from build123d import *

# Parameters (mm, degrees)
ESQUISSE2_R                  = 14.25
BOSS_EXTRU_1_DEPTH           = 3.25
ESQUISSE3_R                  = 1.2
ENL_V_MAT_EXTRU_1_DEPTH      = 4.25
ESQUISSE10_R                 = 1.7
ENL_V_MAT_EXTRU_2_DEPTH      = 1
ENL_V_MAT_EXTRU_2_DEPTH_BACK = 7.5
ESQUISSE17_R                 = 4
ENL_V_MAT_EXTRU_8_DEPTH      = 2
ESQUISSE13_R                 = 1
ENL_V_MAT_EXTRU_4_DEPTH      = 35.402543264


with BuildPart() as part:
    # Esquisse2 → Boss.-Extru.1 (new body, symmetric)
    with BuildSketch(Plane.XY):
        Circle(ESQUISSE2_R)
    extrude(amount=BOSS_EXTRU_1_DEPTH, both=True)

    # Esquisse3 → Enlèv. mat.-Extru.1 (cut, through all)
    with BuildSketch(Plane.XY):
        with Locations((0, 8.25)):
            Circle(ESQUISSE3_R)
        with Locations((-8.25, 0)):
            Circle(ESQUISSE3_R)
        with Locations((0, -8.25)):
            Circle(ESQUISSE3_R)
        with Locations((8.25, 0)):
            Circle(ESQUISSE3_R)
    extrude(amount=ENL_V_MAT_EXTRU_1_DEPTH, mode=Mode.SUBTRACT)

    # Esquisse10 → Enlèv. mat.-Extru.2 (cut, two sides)
    with BuildSketch(Plane(origin=(0, 0, -3.25), x_dir=(-1, 0, 0), z_dir=(0, 0, -1))) as enl_v_mat_extru_2_sk:
        with Locations((-8.25, 0)):
            Circle(ESQUISSE10_R)
        with Locations((0, 8.25)):
            Circle(ESQUISSE10_R)
        with Locations((8.25, 0)):
            Circle(ESQUISSE10_R)
        with Locations((0, -8.25)):
            Circle(ESQUISSE10_R)
    extrude(amount=ENL_V_MAT_EXTRU_2_DEPTH, mode=Mode.SUBTRACT)
    extrude(enl_v_mat_extru_2_sk.sketch, amount=-ENL_V_MAT_EXTRU_2_DEPTH_BACK, mode=Mode.SUBTRACT)

    # Esquisse17 → Enlèv. mat.-Extru.8 (cut)
    with BuildSketch(Plane.XY.offset(3.25)):
        Circle(ESQUISSE17_R)
    extrude(amount=-ENL_V_MAT_EXTRU_8_DEPTH, mode=Mode.SUBTRACT)

    # Esquisse13 → Enlèv. mat.-Extru.4 (cut, through all)
    with BuildSketch(Plane(origin=(10.076271632, -10.076271632, 0), x_dir=(-0.707106781, -0.707106781, 0), z_dir=(0.707106781, -0.707106781, 0))):
        Circle(ESQUISSE13_R)
    extrude(amount=-ENL_V_MAT_EXTRU_4_DEPTH, mode=Mode.SUBTRACT)

    # Esquisse18 → Enlèvement de matière-Révolution1 (revolve, cut)
    with BuildSketch(Plane(origin=(0, 0, 0), x_dir=(1, 0, 0), z_dir=(0, 1, 0))):
        Polygon((14.25, 2.5), (12.806624327, 0), (14.25, -2.5), align=None)
    revolve(axis=Axis((0, 0, -3.25), (0, 0, 1)), mode=Mode.SUBTRACT)


solid = part.part
Design review of the part built by this model. Coordinates are the model's own, in mm. A direction names the side the tool comes from. Give positions to 0.01 mm unless a question says otherwise; leave off trailing zeros. Order: outer loops, then holes, each group sorted by start corner. A loop starts at its lowest first (then second) coordinate and runs counter-clockwise, first axis right, second up.
1. Mouldability with a two-part tool opening along Y and no side actions: class faces 1 (the cylindrical face through (13.163, -5.458, 2.88)), 2 (the cylindrical face through (0.37, 6.59, -0.05)), 3 (the cylindrical face through (-0.54, -0.81, -0.3)), 4 (the flat face through (0, 0, -3.25)) as +Y half, -Y half, draft (parallel to the pull), parting line (faces both ways), or undercut.
Solution:
face 1: parting line
face 2: undercut
face 3: undercut
face 4: draft
2. To check wall thickness, follow L1, parallel to Y at x = 0, z = 2.65; L2, parallel to Y at x = -8.5, z = 0.5; L3, parallel to Y at x = -9, z = 1.5. State the ranges of each line that lie inside material, in increasing order.
Solution:
L1: y = -14.25 to -9.95, -6.55 to -4, 4 to 6.55, 9.95 to 14.25
L2: y = -9.96 to -1.68, 1.68 to 7.28, 9.72 to 9.96
L3: y = -10.29 to -1.53, 1.53 to 10.29
3. Tool access review of faces 5 (the flat face through (0, 0, 1.25)), 6 (the cylindrical face through (-6.9, -1.03, -0.05)), 7 (the conical face through (6.016, -11.566, -0.399)): name each direction out of +Z, -Z, +X, -X, +Y, -Y from which nothing blocks a thin tool from reaching the whole face with its end or side.
Solution:
face 5: +Z
face 6: +Z, -Z
face 7: none
4. For pin 1 Ø3 at (x, z) = (-10.5, -1) entering from -Y; pin 2 Ø1 at (y, z) = (-8, 0) entering from +X; pin 3 Ø1 at (x, z) = (-8.5, -1) entering from -Y, all flat-tipped, find the tip position at first contact; note any pin that passes through.
Solution:
pin 1: stops at y = -10.34
pin 2: stops at x = 10.53
pin 3: stops at y = -10.88
5. Add section D-D, the plane z = 2. State the section outline as (x, y) points, then the cut area to 3 significant figures.
Solution:
outline: circle Ø27.92 at (0, 0); hole circle Ø3.4 at (-8.25, 0); hole circle Ø8 at (0, 0); hole circle Ø3.4 at (0, -8.25); hole circle Ø3.4 at (0, 8.25); hole circle Ø3.4 at (8.25, 0)
area: 526 mm2
6. Add section A-A, the plane z = -0.5. State the section outline as (x, y) points.
Solution:
outline: (-9.85, 8.63) arc R13.1 ccw to (8.63, -9.85) - close; (-8.63, 9.85) - (9.85, -8.63) arc R13.1 ccw to start; hole circle Ø3.4 at (-8.25, 0); hole circle Ø3.4 at (0, -8.25); hole circle Ø3.4 at (0, 8.25); hole circle Ø3.4 at (8.25, 0)
7. Add section B-B, the plane x = 0. State how many separate pieces and enclosed holes the cut face has, then the cut area to 3 significant figures.
Solution:
separate pieces: 3
enclosed holes: 1
area: 113 mm2
